Autodesk Fusion 360 part; units mm, degrees
sketch "Esboço1" plane through (0, 0, 0) normal (0, 1, 0) x (1, 0, 0)
  circle A0 centre (0, 0) radius 4.5
  circle A1 centre (0, 0) radius 1.5
  dimension "d1" = 9
  dimension "d2" = 3
extrude "Extrusão1" add sketch "Esboço1" along normal blind 1.5
extrude "Extrusão2" cut 1 faces at (3.4832, 1.5, 0.2236) along direction (0, -1, 0) blind 0.7
extrude "Extrusão3" add 1 faces at (3.4832, 0.8, 0.2236) along direction (0, 1, 0) blind 0.2
Geometry check sheet. Reference: the model listing, model coordinates, mm. Round coordinates to 2 decimals unless told otherwise and drop trailing zeros. Loops run counter-clockwise (first coordinate to the right, second up) from the corner with the lowest first, then second, coordinate; pieces in that order, holes last. Notation, with made-up numbers: M 17.25,43 L 54.25,43 A19 cw 54.25,65 Z; hole C -8,-16.75 d6. An arc over 180 degrees is marked long. Return JSON: item names as keys, results as strings. Group by question number.
(1) Scan lines: line 1 along X through (y, z) = (0.55, 0); line 2 along X through (y, z) = (0.25, 0.5). Record each from-to range of solid material in increasing order. Write a range as [from, to].
(2) Section check D-D, the plane z = -2. Enter the section's corners in (x, y).
(3) Section check C-C, the plane y = 0.6. Enter the section's corners in (x, z), and give its area (3 significant figures).
(4) Section check B-B, the plane x = 0. Enter the section's corners in (y, z), and give its area (3 significant figures).
(5) Section check A-A, the plane z = 0. Enter the section's corners in (x, y), and give its area (3 significant figures).
(6) Go/stop test with a flat-tipped pin: pin 1 (5 mm diameter, centred on x = 0, z = 0, fed in from +Y). Record where the tip stops, or that it passes through.
(7) Mould release check, pull along Z, two halves, no side actions. Record for faces 1 (the face through (-0.59, 0.49, 4.46)), 2 (the face through (-1.5, 0.49, 0.07)), 3 (the face through (0, 1, 2)): pulls with the +Z half, pulls with the -Z half, needs draft (parallel to the pull), parting line crosses it, or undercut.
Data:
{
 "1": {"line 1": "[-4.5, -1.5], [1.5, 4.5]", "line 2": "[-4.47, -1.41], [1.41, 4.47]"},
 "2": {"outline": "M -4.03,0 L 4.03,0 L 4.03,1 L -4.03,1 Z"},
 "3": {"outline": "C 0,0 d9; hole C 0,0 d3", "area": "56.5 mm²"},
 "4": {"outline": "M 0,-4.5 L 1,-4.5 L 1,-1.5 L 0,-1.5 Z; M 0,1.5 L 1,1.5 L 1,4.5 L 0,4.5 Z", "area": "6.00 mm²"},
 "5": {"outline": "M -4.5,0 L -1.5,0 L -1.5,1 L -4.5,1 Z; M 1.5,0 L 4.5,0 L 4.5,1 L 1.5,1 Z", "area": "6.00 mm²"},
 "6": {"pin 1": "y = 1"},
 "7": {"face 1": "parting line crosses it", "face 2": "undercut", "face 3": "needs draft"}
}
